from build123d import *

# Parameters (mm, degrees)
BASE_FLANGE1_DEPTH      = 100
SKETCH8_W               = 29
SKETCH8_H               = 12
SKETCH8_R               = 3
CUT_EXTRUDE1_DEPTH      = 159.28139499
CUT_EXTRUDE2_DEPTH      = 157.74501587
CUT_EXTRUDE2_DEPTH_BACK = 157.74501587
CUT_EXTRUDE4_START      = -2
CUT_EXTRUDE4_OUTLINE_W  = 3
CUT_EXTRUDE4_OUTLINE_H  = 58
CUT_EXTRUDE4_DEPTH      = 3
CUT_EXTRUDE5_DEPTH      = 157.74501587
CUT_EXTRUDE5_DEPTH_BACK = 157.74501587
SKETCH11_W              = 50
SKETCH11_H              = 58
CUT_EXTRUDE6_DEPTH      = 157.74501587
CUT_EXTRUDE6_DEPTH_BACK = 157.74501587
SKETCH12_R              = 2.5


# Read off the part's stored shape, not the designer's step: Cut-Extrude4
# Sheet-metal steps are written as plain solids
with BuildPart() as part:
    # Sketch1 → Base-Flange1 (new body)
    with BuildSketch(Plane.XY):
        with BuildLine():
            Line((0, 13), (0, 1))
            ThreePointArc((0, 1), (0.292893219, 0.292893219), (1, 0))
            Line((1, 0), (120, 0))
            Line((120, 0), (120, -2))
            Line((120, -2), (1, -2))
            ThreePointArc((1, -2), (-1.121320344, -1.121320344), (-2, 1))
            Line((-2, 1), (-2, 13))
            Line((-2, 13), (0, 13))
        make_face()
    extrude(amount=BASE_FLANGE1_DEPTH)

    # Sketch8 → Cut-Extrude1 (cut, through all)
    with BuildSketch(Plane.ZY.offset(2)):
        with Locations((35.5, 7)):
            Rectangle(SKETCH8_W, SKETCH8_H)
        with Locations((64.5, 7)):
            Rectangle(SKETCH8_W, SKETCH8_H)
        with Locations((10.5, 7)):
            Circle(SKETCH8_R)
        with Locations((89.5, 7)):
            Circle(SKETCH8_R)
    extrude(amount=-CUT_EXTRUDE1_DEPTH, mode=Mode.SUBTRACT)

    # Sketch9 → Cut-Extrude2 (cut, two sides: drawn at the far end of the back side and taken through both)
    with BuildSketch(Plane(origin=(0, 0, 0), x_dir=(1, 0, 0), z_dir=(0, 1, 0)).offset(-CUT_EXTRUDE2_DEPTH_BACK)):
        with BuildLine():
            Line((112, -10), (112, -90))
            ThreePointArc((112, -90), (110, -92), (108, -90))
            Line((108, -90), (108, -10))
            ThreePointArc((108, -10), (110, -8), (112, -10))
        make_face()
        with BuildLine():
            Line((93, -10), (93, -90))
            ThreePointArc((93, -90), (95, -92), (97, -90))
            Line((97, -90), (97, -10))
            ThreePointArc((97, -10), (95, -8), (93, -10))
        make_face()
    extrude(amount=CUT_EXTRUDE2_DEPTH + CUT_EXTRUDE2_DEPTH_BACK, mode=Mode.SUBTRACT)

    # Cut-Extrude4 outline → Cut-Extrude4 (cut)
    with BuildSketch(Plane(origin=(0, 0, 0), x_dir=(1, 0, 0), z_dir=(0, 1, 0)).offset(CUT_EXTRUDE4_START)):
        with Locations((-0.5, -50)):
            Rectangle(CUT_EXTRUDE4_OUTLINE_W, CUT_EXTRUDE4_OUTLINE_H)
    extrude(amount=CUT_EXTRUDE4_DEPTH, mode=Mode.SUBTRACT)

    # Sketch11 → Cut-Extrude5 (cut, two sides: drawn at the far end of the back side and taken through both)
    with BuildSketch(Plane(origin=(0, 0, 0), x_dir=(1, 0, 0), z_dir=(0, 1, 0)).offset(-CUT_EXTRUDE5_DEPTH_BACK)):
        with Locations((26, -50)):
            Rectangle(SKETCH11_W, SKETCH11_H)
    extrude(amount=CUT_EXTRUDE5_DEPTH + CUT_EXTRUDE5_DEPTH_BACK, mode=Mode.SUBTRACT)

    # Sketch12 → Cut-Extrude6 (cut, two sides: drawn at the far end of the back side and taken through both)
    with BuildSketch(Plane(origin=(0, 0, 0), x_dir=(1, 0, 0), z_dir=(0, 1, 0)).offset(-CUT_EXTRUDE6_DEPTH_BACK)):
        with Locations(Location((21, -10.5, 0), (0, 0, 270))):
            Circle(SKETCH12_R)
        with Locations(Location((41, -10.5, 0), (0, 0, 270))):
            Circle(SKETCH12_R)
        with Locations(Location((21, -89.5, 0), (0, 0, 270))):
            Circle(SKETCH12_R)
        with Locations(Location((41, -89.5, 0), (0, 0, 270))):
            Circle(SKETCH12_R)
        with Locations(Location((76, -89.5, 0), (0, 0, 270))):
            Circle(SKETCH12_R)
        with Locations(Location((56, -89.5, 0), (0, 0, 270))):
            Circle(SKETCH12_R)
        with Locations(Location((56, -10.5, 0), (0, 0, 270))):
            Circle(SKETCH12_R)
        with Locations(Location((76, -10.5, 0), (0, 0, 270))):
            Circle(SKETCH12_R)
    extrude(amount=CUT_EXTRUDE6_DEPTH + CUT_EXTRUDE6_DEPTH_BACK, mode=Mode.SUBTRACT)


solid = part.part
Build history of the part. All positions in model axes, mm. Give positions to 0.01 mm unless a question says otherwise; leave off trailing zeros. Order: outer loops, then holes, each group sorted by start corner. A loop starts at its lowest first (then second) coordinate and runs counter-clockwise, first axis right, second up. Notation, with made-up numbers: M 88.25,37 L 119.25,37 A18 cw 119.25,70 Z; hole C -1.75,-24 d2. An arc over 180 degrees is marked long. Use one line per item in the form item = value.
1) Saw through at B-B (x = 15.5). Give the cut face in (y, z).
Calculated:
outline = M -2,0 L 0,0 L 0,21 L -2,21 Z; M -2,79 L 0,79 L 0,100 L -2,100 Z
2) Saw through at D-D (x = 56). Give the cut face in (y, z), plus the area to 3 significant figures.
Calculated:
outline = M -2,0 L 0,0 L 0,8 L -2,8 Z; M -2,13 L 0,13 L 0,87 L -2,87 Z; M -2,92 L 0,92 L 0,100 L -2,100 Z
area = 180 mm2
3) Saw through at C-C (z = 35.5). Give the cut face in (x, y), plus the area to 3 significant figures.
Calculated:
outline = M 51,-2 L 93,-2 L 93,0 L 51,0 Z; M 97,-2 L 108,-2 L 108,0 L 97,0 Z; M 112,-2 L 120,-2 L 120,0 L 112,0 Z
area = 122 mm2
4) Two-plate mould, pull along Z, no slides. Class faces 1 (the face through (0, 10, 92)), 2 (the face through (-1.01, 9.53, 12.11)), 3 (the face through (59, -1, 0)), 4 (the face through (20, -1, 79)): released by +Z, released by -Z, zero draft, split by the parting line, or undercut.
Calculated:
face_1 = zero draft
face_2 = undercut
face_3 = released by -Z
face_4 = undercut
5) Saw through at A-A (x = 41). Give the cut face in (y, z).
Calculated:
outline = M -2,0 L 0,0 L 0,8 L -2,8 Z; M -2,13 L 0,13 L 0,21 L -2,21 Z; M -2,79 L 0,79 L 0,87 L -2,87 Z; M -2,92 L 0,92 L 0,100 L -2,100 Z
6) Probe probe 1 along Z at (x, y) = (56, -1.5); probe 2 along X at (y, z) = (-0.5, 27.5); probe 3 along Z at (x, y) = (41, -1.3). List the from-to ranges inside material, lowest first.
Calculated:
probe_1 = 0 to 8, 13 to 87, 92 to 100
probe_2 = 51 to 93, 97 to 108, 112 to 120
probe_3 = 0 to 8, 13 to 21, 79 to 87, 92 to 100
7) Drop flat-ended pins along their axis: pin 1 (1 mm diameter, centred on y = -1, z = 41, fed in from -X); pin 2 (8 mm diameter, centred on x = 76, z = 10.5, fed in from +Y); pin 3 (3 mm diameter, centred on x = 21, z = 89.5, fed in from -Y); pin 4 (3.5 mm diameter, centred on y = 4.5, z = 87, fed in from +X). Give the stop position or say it passes through.
Calculated:
pin_1 = 51
pin_2 = 0
pin_3 = through
pin_4 = 0
